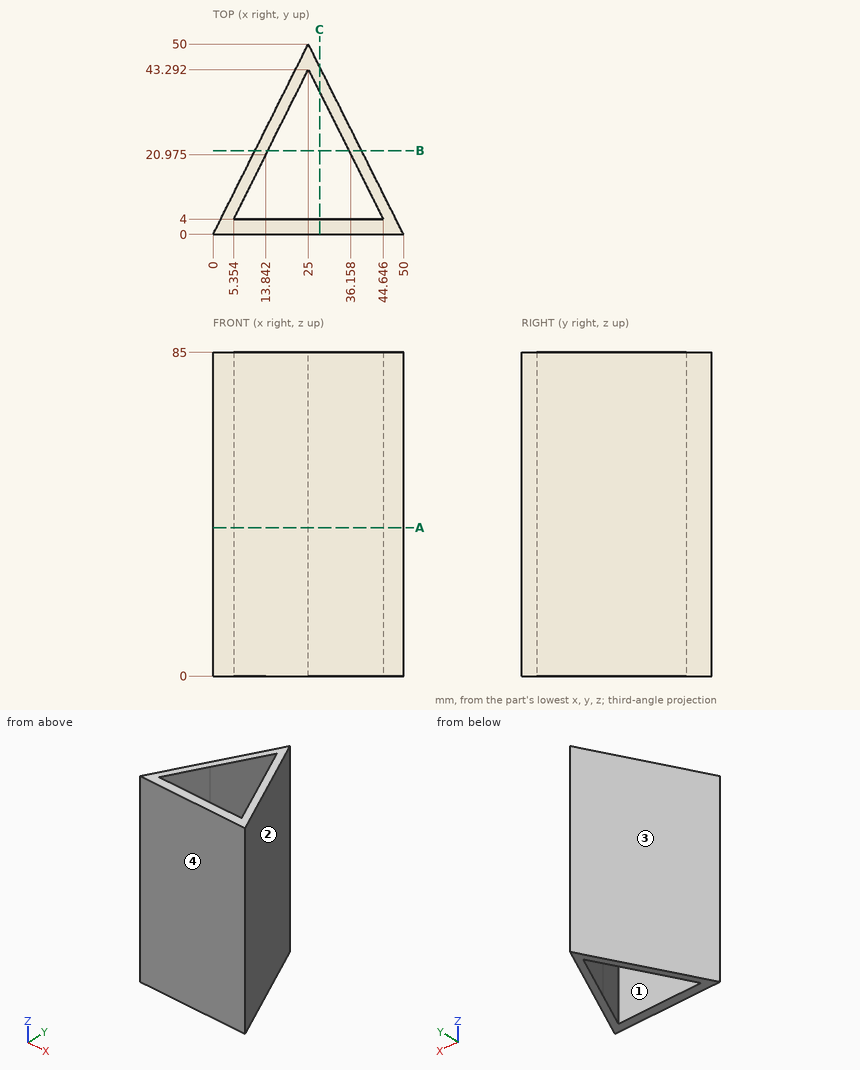
Answer from the drawing. Dimensions are ordinates in mm from the lowest x, y and z of the part. Give positions to 0.01 mm unless a question says otherwise; leave off trailing zeros. Order: outer loops, then holes, each group sorted by start corner. A loop starts at its lowest first (then second) coordinate and runs counter-clockwise, first axis right, second up. Notation, with made-up numbers: (67, 54) - (123, 54) arc R27 cw to (123, 76) - close; hole circle Ø1 at (37.25, 51.5). An arc over 180 degrees is marked (long way). Use one line per item in the form item = value.
1) Find section B-B on y = 22. Determine the outline of the cut face in (x, z).
Verdict:
outline = (11, 0) - (14.35, 0) - (14.35, 85) - (11, 85) - close; (35.65, 0) - (39, 0) - (39, 85) - (35.65, 85) - close
2) Find section C-C on x = 28. Determine the outline of the cut face in (y, z).
Verdict:
outline = (0, 0) - (4, 0) - (4, 85) - (0, 85) - close; (37.29, 0) - (44, 0) - (44, 85) - (37.29, 85) - close
3) Each of these flat-tipped pins is pushed along its axis until it touches: pin 1 (5 mm diameter, centred on y = 12.5, z = 28.5, fed in from -X); pin 2 (1 mm diameter, centred on x = 16, z = 30, fed in from +Y); pin 3 (10 mm diameter, centred on y = 41, z = 10, fed in from -X). Where does it stop, or does it pass through?
Verdict:
pin_1 = 5
pin_2 = 33
pin_3 = 18
4) Find section A-A on z = 39. Determine the outline of the cut face in (x, y) (1 decimal).
Verdict:
outline = (0, 0) - (50, 0) - (25, 50) - close; hole (5.4, 4) - (44.6, 4) - (36.2, 21) - (25, 43.3) - (13.8, 21) - close
5) Consider probe 1 along Y at (x, z) = (11.5, 59) (1 decimal); probe 2 along Y at (x, z) = (26, 78.5) (1 decimal); probe 3 along X at (y, z) = (26, 5.5) (1 decimal). Determine where each line is inside the solid, lowest interval first. Write a range as [from, to].
Verdict:
probe_1 = [0, 4], [16.3, 23]
probe_2 = [0, 4], [41.3, 48]
probe_3 = [13, 16.4], [33.6, 37]
6) The mould has two halves that part along X. Classify the marked faces 1, 2, 3 and 4: released by +X, released by -X, zero draft, split by the parting line, or undercut.
Verdict:
face_1 = undercut
face_2 = released by +X
face_3 = released by -X
face_4 = zero draft
